Input: part model. Units: mm. Frame: model coordinates. Round coordinates to 2 decimals unless told otherwise and drop trailing zeros. Order: outer loops, then holes, each group sorted by start corner. A loop starts at its lowest first (then second) coordinate and runs counter-clockwise, first axis right, second up. Notation, with made-up numbers: (-32.75, 82) -> (-4.75, 82) arc R8 ccw to (-4.75, 90) -> close; hole circle Ø10 at (72, 71.5). An arc over 180 degrees is marked (long way). Use a Markdown table: item, result.
from build123d import *

# Parameters (mm, degrees)
F0_R           = 5
F0_R_2         = 20
F1_DEPTH       = 6
F3_D           = 6.6
F4_D           = 4.5
F4_CSINK_D     = 8.96
F4_CSINK_ANGLE = 90
F5_D           = 5.5
F5_CSINK_D     = 11.2
F5_CSINK_ANGLE = 90
F6_D           = 4
F7_D           = 8
F8_D           = 5
F10_D          = 2.5
F10_DEPTH      = 5
F10_TIP        = 0.7510757738


with BuildPart() as f1:
    # F0 (on Front) → F1 (new body)
    with BuildSketch(Plane.XZ):
        with BuildLine():
            Line((-116.6983369343, 12), (-125.8983369343, 12))
            ThreePointArc((-125.8983369343, 12), (-137.8983369343, 0), (-125.8983369343, -12))
            Line((-125.8983369343, -12), (-116.6983369343, -12))
            ThreePointArc((-116.6983369343, -12), (-111.5765110931, -13.4112340786), (-107.9003042862, -17.2466199896))
            ThreePointArc((-107.9003042862, -17.2466199896), (-89.6210681696, -41.3493023164), (-60.7881962998, -50.5))
            Line((-60.7881962998, -50.5), (-29.6183369343, -50.5))
            Line((-29.6183369343, -50.5), (94.1016630657, -50.5))
            ThreePointArc((94.1016630657, -50.5), (101.1727308776, -47.5710678119), (104.1016630657, -40.5))
            Line((104.1016630657, -40.5), (104.1016630657, 40.5))
            ThreePointArc((104.1016630657, 40.5), (101.1727308776, 47.5710678119), (94.1016630657, 50.5))
            Line((94.1016630657, 50.5), (-60.7881962998, 50.5))
            ThreePointArc((-60.7881962998, 50.5), (-89.6210681696, 41.3493023164), (-107.9003042862, 17.2466199896))
            ThreePointArc((-107.9003042862, 17.2466199896), (-111.5765110931, 13.4112340786), (-116.6983369343, 12))
        make_face()
        with Locations((-125.8983369343, 0)):
            Circle(F0_R, mode=Mode.SUBTRACT)
        with Locations((37.1016630657, 0)):
            Circle(F0_R_2, mode=Mode.SUBTRACT)
    extrude(amount=F1_DEPTH)

    # F3 (through all)
    with Locations(Plane.XZ.offset(6)):
        with Locations((1.2016630657, 44.8), (-20.1483369343, 44.8)):
            Hole(F3_D / 2)

    # F4 (through all)
    with Locations(Plane.XZ.offset(6)):
        with Locations((2.3016630657, 36), (11.2016630657, 38)):
            CounterSinkHole(F4_D / 2, F4_CSINK_D / 2, counter_sink_angle=F4_CSINK_ANGLE)

    # F5 (through all)
    with Locations(Plane.XZ.offset(6)):
        with Locations((19.1016630657, 23.5), (92.1016630657, 23.5), (92.1016630657, -23.5), (19.1016630657, -23.5), (-35.1783369343, -23.2), (-24.9183369343, 1.7480218202), (-54.0483369343, 15.6), (-64.3083369343, -9.3480218202)):
            CounterSinkHole(F5_D / 2, F5_CSINK_D / 2, counter_sink_angle=F5_CSINK_ANGLE)

    # F6 (through all)
    with Locations(Plane.XZ.offset(6)):
        with Locations((37.1016630657, -42.9)):
            Hole(F6_D / 2)

    # F7 (through all)
    with Locations(Plane.XZ.offset(6)):
        with Locations((70.1016630657, 18.5), (70.1016630657, -18.5), (-30.0483369343, -9.1), (-59.1783369343, 1.52)):
            Hole(F7_D / 2)

    # F8 (through all)
    with Locations(Plane.XZ.offset(6)):
        with Locations((2.1016630657, -20)):
            Hole(F8_D / 2)

    # F10
    with Locations(Plane.XY.offset(50.5)):
        with Locations((49.0775220096, -3), (-35.9050817788, -3)):
            Hole(F10_D / 2, depth=F10_DEPTH)
            with Locations((0, 0, -(F10_DEPTH + F10_TIP / 2))):  # 118° drill point
                Cone(0, F10_D / 2, F10_TIP, mode=Mode.SUBTRACT)


solid = f1.part
1) Line query: L1, parallel to X at y = -3.9, z = -17; L2, parallel to X at y = -5, z = -9.5; L3, parallel to Z at x = 72, y = -1.3. Output: solid intervals per line, ascending. Write a range as [from, to].
Results found:
| item | result |
|---|---|
| L1 | x = [-108.04, 26.57], [47.64, 66.39], [73.81, 104.1] |
| L2 | x = [-133.23, -68.91], [-59.71, -34.03], [-26.07, 19.5], [54.7, 104.1] |
| L3 | z = [-50.5, -22.02], [-14.98, 14.98], [22.02, 50.5] |
2) Cut plane A-A on x = -83. Return loops of the section in (y, z), and give its area (3 significant figures).
Results found:
| item | result |
|---|---|
| outline | (-6, -45.3) -> (0, -45.3) -> (0, 45.3) -> (-6, 45.3) -> close |
| area | 544 mm² |
3) Pin query (flat end, axial travel): pin 1 Ø1 at (x, y) = (-102.5, -3.5) entering from +Z; pin 2 Ø3 at (x, y) = (-94, -5) entering from +Z. Return the tip coordinate at first contact, or that it passes through.
Results found:
| item | result |
|---|---|
| pin 1 | stops at z = 28.81 |
| pin 2 | stops at z = 39.16 |
4) Pull-direction query (Z, two-part tool) for faces 1 (the cylindrical face through (-111.51, -2.96, 13.45)), 2 (the cylindrical face through (56.178, -2.958, 6.007)), 3 (the cylindrical face through (101.095, -2.958, -47.648)); classes: +Z half, -Z half, draft (parallel to the pull), parting line (faces both ways), or undercut.
Results found:
| item | result |
|---|---|
| face 1 | +Z half |
| face 2 | undercut |
| face 3 | -Z half |
